For this review, take the finished solid that the model builds, in its own axes (mm). A direction names the side the tool comes from. Give positions to 0.01 mm unless a question says otherwise; leave off trailing zeros. Order: outer loops, then holes, each group sorted by start corner. A loop starts at its lowest first (then second) coordinate and runs counter-clockwise, first axis right, second up. Notation, with made-up numbers: (19, 40) - (69, 40) arc R28 ccw to (69, 70) - close; hole circle Ø4 at (-7, 11.5). An arc over 180 degrees is marked (long way). Use a Markdown table: item, result. Add a question column.
1) Wall thickness on L1, parallel to Y at x = 0, z = 2; L2, parallel to Y at x = 2, z = 5; L3, parallel to X at y = 17, z = -0.5: over which ranges is each line inside the solid? List them lowest first.
2) Machinability: for faces 1 (the face through (0, 33, 0)), 2 (the face through (0.45, 30.48, 1.43)), which of the approach directions +Z, -Z, +X, -X, +Y, -Y give a long, thin tool a straight path to every point of the face, cutting with its end or side? Answer none if there is none.
3) We need section C-C on y = 17. Write out the cut boundary in (x, z), then the cut area to 3 significant figures.
4) Mouldability with a two-part tool opening along Y and no side actions: class faces 3 (the face through (0, 25, 6)), 4 (the face through (-1.908, 16.399, -0.042)), 5 (the face through (3, 26, 5)) as released by +Y, released by -Y, zero draft, split by the parting line, or undercut.
5) We need section B-B on y = 10.5. Write out the cut boundary in (x, z), then the cut area to 3 significant figures.
6) We need section A-A on z = 4.75. Write out the cut boundary in (x, y).
7) Clearance check with flat-ended pins moving along their axes: P1, Ø1.2, axis at x = -0.5, z = 4, coming from the +Y side; P2, Ø1.5, axis at x = 0, y = 15.5, coming from the +Z side. State where each tip first meets the part, or that it passes through.
```python
from build123d import *

# Parameters (mm, degrees)
SKETCH2_R               = 3
BOSS_EXTRUDE1_DEPTH     = 25
BOSS_EXTRUDE2_DEPTH     = 4
SKETCH5_R               = 3
BOSS_EXTRUDE3_DEPTH     = 4
FILLET1_R               = 1
CUT_EXTRUDE1_DEPTH      = 4
CUT_EXTRUDE1_DEPTH_BACK = 4
SKETCH6_R               = 2
SKETCH7_R               = 1.5
BOSS_EXTRUDE4_DEPTH     = 4
FILLET2_R               = 1
BOSS_EXTRUDE5_START     = 1.5
SKETCH8_R               = 3
BOSS_EXTRUDE5_DEPTH     = 1.5


with BuildPart() as part:
    # Sketch2 → Boss-Extrude1 (new body)
    with BuildSketch(Plane(origin=(0, 0, 0), x_dir=(1, 0, 0), z_dir=(0, 1, 0))):
        with Locations(Location((0, 0, 0), (0, 0, 270))):
            Circle(SKETCH2_R)
    extrude(amount=BOSS_EXTRUDE1_DEPTH)



with BuildPart() as body_2:
    # Sketch4 → Boss-Extrude2 (new body)
    with BuildSketch(Plane(origin=(0, 25, 0), x_dir=(1, 0, 0), z_dir=(0, 1, 0))):
        with BuildLine():
            Line((-3, 0), (-3, -10))
            Line((-3, -10), (3, -10))
            Line((3, -10), (3, 0))
            ThreePointArc((3, 0), (0, -3), (-3, 0))
        make_face()
    extrude(amount=BOSS_EXTRUDE2_DEPTH)


with BuildPart() as part_1:
    add(part.part)

    add(body_2.part)  # Boss-Extrude3 merges body 2
    # Sketch5 → Boss-Extrude3 (add)
    with BuildSketch(Plane(origin=(0, 25, 0), x_dir=(1, 0, 0), z_dir=(0, 1, 0))):
        Circle(SKETCH5_R)
    extrude(amount=BOSS_EXTRUDE3_DEPTH)

    # Fillet1
    fillet1_edges = [part_1.edges().sort_by_distance(p)[0] for p in [
        (0, 29, -3),
        (3, 27, 10),
        (-3, 27, 10),
        (3, 29, 5),
        (-3, 29, 5),
        (0, 29, 10),
    ]]
    fillet(fillet1_edges, radius=FILLET1_R)

    # Sketch6 → Cut-Extrude1 (cut, two sides: drawn at the far end of the back side and taken through both)
    with BuildSketch(Plane.XY.offset(-CUT_EXTRUDE1_DEPTH_BACK)):
        with Locations(Location((0, 17, 0), (0, 0, 180))):
            Circle(SKETCH6_R)
    extrude(amount=CUT_EXTRUDE1_DEPTH + CUT_EXTRUDE1_DEPTH_BACK, mode=Mode.SUBTRACT)

    # Sketch7 → Boss-Extrude4 (add)
    with BuildSketch(Plane(origin=(0, 29, 0), x_dir=(1, 0, 0), z_dir=(0, 1, 0))):
        with Locations(Location((0, 0, 0), (0, 0, 270))):
            Circle(SKETCH7_R)
    extrude(amount=BOSS_EXTRUDE4_DEPTH)

    # Fillet2
    fillet2_edges = [part_1.edges().sort_by_distance(p)[0] for p in [
        (0, 33, -1.5),
    ]]
    fillet(fillet2_edges, radius=FILLET2_R)

    # Sketch8 → Boss-Extrude5 (add)
    with BuildSketch(Plane(origin=(0, 0, 0), x_dir=(-1, 0, 0), z_dir=(0, -1, 0)).offset(BOSS_EXTRUDE5_START)):
        with Locations(Location((0, 0, 0), (0, 0, 90))):
            Circle(SKETCH8_R)
    extrude(amount=-BOSS_EXTRUDE5_DEPTH)


solid = part_1.part
```
Checked values:
| question | item | result |
|---|---|---|
| 1 | L1 | -1.5 to 15, 19 to 29 |
| 1 | L2 | 25 to 29 |
| 1 | L3 | -2.96 to -2, 2 to 2.96 |
| 2 | face 1 | +Z, -Z, +X, -X, +Y |
| 2 | face 2 | +Y |
| 3 | outline | (-2, -2.24) - (-2, 2.24) arc R3 ccw to start; (2, -2.24) arc R3 ccw to (2, 2.24) - close |
| 3 | area | 6.19 mm² |
| 4 | face 3 | released by -Y |
| 4 | face 4 | undercut |
| 4 | face 5 | zero draft |
| 5 | outline | circle Ø6 at (0, 0) |
| 5 | area | 28.3 mm² |
| 6 | outline | (-3, 25) - (3, 25) - (3, 28) arc R1 ccw to (2, 29) - (-2, 29) arc R1 ccw to (-3, 28) - close |
| 7 | P1 | y = 29 |
| 7 | P2 | z = 3 |
